from build123d import *

# Parameters (mm, degrees)
SKETCH1_R           = 2.75
BOSS_EXTRUDE1_DEPTH = 20
SKETCH2_R           = 4
BOSS_EXTRUDE2_DEPTH = 2
FILLET1_SIZE        = 2
FILLET1_SIZE_2      = 1


with BuildPart() as part:
    # Sketch1 → Boss-Extrude1 (new body)
    with BuildSketch(Plane(origin=(0, 0, 0), x_dir=(0, 0, -1), z_dir=(1, 0, 0))):
        Circle(SKETCH1_R)
    extrude(amount=BOSS_EXTRUDE1_DEPTH)

    # Sketch2 → Boss-Extrude2 (add)
    with BuildSketch(Plane.ZY):
        Circle(SKETCH2_R)
    extrude(amount=BOSS_EXTRUDE2_DEPTH)

    # Fillet1
    # an asymmetric fillet: 2, 1 mm, written as the material it takes off along each edge
    with BuildSketch(Plane(origin=(-2, 0, 0), x_dir=(0, 0, 1), z_dir=(0, -1, 0))) as fillet1_piece_1:
        with BuildLine():
            Bezier((4, -FILLET1_SIZE), (4, 0), (4 - FILLET1_SIZE_2, 0), weights=[1, 0.707106781, 1])
            Line((4 - FILLET1_SIZE_2, 0), (4, 0))
            Line((4, 0), (4, -FILLET1_SIZE))
        make_face()
    revolve(axis=Axis((-2, 0, 0), (-1, 0, 0)), mode=Mode.SUBTRACT)


solid = part.part
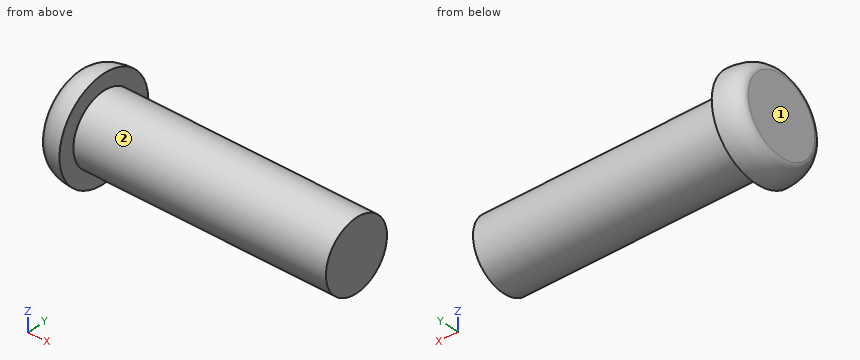
Input: part model. Units: mm. Frame: model coordinates. Face numbers are marked on the shaded views. A direction names the side the tool comes from. Round coordinates to 2 decimals unless told otherwise and drop trailing zeros. Write each loop counter-clockwise with the first axis right and the second up, starting at its lowest first coordinate (ties: lowest second). Pieces come first, ordered by that corner, then holes.
1) Cut plane A-A (x = 9.5). Return the cut outline in (y, z), then the cut area to 3 significant figures.
2) Ray query, L1, parallel to X at y = -0.5, z = 3; L2, parallel to Y at x = 9.75, z = 1.5; L3, parallel to Z at x = 8.5, y = 2. Return the intervals inside material, ascending.
3) Reachability of the marked faces 1 and 2 from +Z, -Z, +X, -X, +Y, -Y: full face, straight path, thin tool, end or side. Return the list, or none.
4) Contact query for flat-ended pins moving along their axis: P1, Ø2, axis at x = 8.5, y = 1, coming from the -Z side; P2, Ø1.5, axis at x = 7.5, z = 2, coming from the -Y side; P3, Ø1, axis at x = 3, z = 3, coming from the +Y side. Output: stop coordinate, or through.
Geometry says:
1. outline: circle Ø5.5 at (0, 0)
1. area: 23.8 mm2
2. L1: x = -2 to 0
2. L2: y = -2.3 to 2.3
2. L3: z = -1.89 to 1.89
3. face 1: +Z, -Z, -X, +Y, -Y
3. face 2: +X
4. P1: stops at z = -2.75
4. P2: stops at y = -2.45
4. P3: stops at y = 1.15
